Could you check a few things on this model? Use its own coordinates, in mm. Face numbers are marked on the shaded views. A direction names the side the tool comes from. Give positions to 0.01 mm unless a question says otherwise; leave off trailing zeros. Loops run counter-clockwise (first coordinate to the right, second up) from the corner with the lowest first, then second, coordinate; pieces in that order, holes last. Notation, with made-up numbers: (-28, 89) -> (11, 89) arc R13 ccw to (11, 96) -> close; hole circle Ø4 at (8.5, 11.25). An arc over 180 degrees is marked (long way). Write item = value, one per line. Start each with the question number.
1) I want a section at B-B (z = 3). List the corners of the cut face in (x, y) for me, and give its area (3 significant figures).
2) On a 3-axis mill with a long thin cutter (end or side, diameter ignored), from which of +Z, -Z, +X, -X, +Y, -Y can I reach the whole of each face in a straight line? I mean the marked faces 1, 2 and 3. Say none if no direction works.
3) I want a section at D-D (z = -32.5). List the corners of the cut face in (x, y) for me.
4) I want a section at A-A (y = -13). List the corners of the cut face in (x, z) for me.
5) I'm going to push flat-ended pins straight in: pin 1 Ø6 at (y, z) = (-9.5, -21.5) entering from +X; pin 2 Ø3 at (x, y) = (27, -13) entering from +Z; pin 3 Ø5 at (x, y) = (-2, -4) entering from +Z; pin 4 Ø4 at (x, z) = (4, -12) entering from +Y. Where does each tip first touch, or does it pass through?
6) If we mould it in two halves opening along X, with no side actions, what happens to the marked faces 4, 5 and 6? For each: +X half, -X half, draft (parallel to the pull), parting line (faces both ways), or undercut.
7) I need wall thicknesses on probe 1 along X at (y, z) = (-1.75, 7.5); probe 2 along Z at (x, y) = (-11, -0.5); probe 3 along Z at (x, y) = (2, -1.25). Which ranges of each line are inside material? Lowest first, please. Write a range as from..to.
8) I want a section at C-C (x = -2). List the corners of the cut face in (y, z) for me, and give its area (3 significant figures).
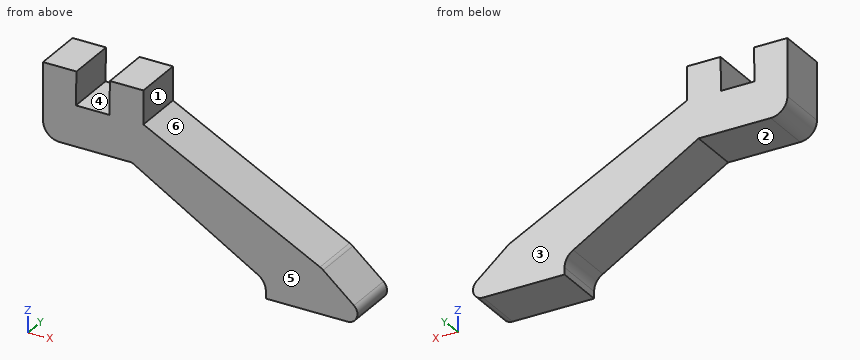
from build123d import *

# Parameters (mm, degrees)
F1_DEPTH = 15
F2_R     = 5


with BuildPart() as f1:
    # F0 (on Front) → F1 (new body)
    with BuildSketch(Plane.XZ):
        with BuildLine():
            Line((65.747503, -27.193502), (12.955731, 0))
            Line((12.955731, 0), (12.955731, 9.998409))
            Line((12.955731, 9.998409), (2.955731, 9.998409))
            Line((2.955731, 9.998409), (2.777357, 0))
            Line((2.777357, 0), (-7.222643, 0))
            Line((-7.222643, 0), (-7.044269, 9.998409))
            Line((-7.044269, 9.998409), (-17.044269, 9.998409))
            Line((-17.044269, 9.998409), (-17.044269, 0))
            Line((-17.044269, 0), (-17.044269, -12.098167))
            Line((-17.044269, -12.098167), (9.505874, -12.098167))
            Line((9.505874, -12.098167), (46.953158, -34.44976))
            ThreePointArc((46.953158, -34.44976), (48.861942, -36.287192), (49.563903, -38.841965))
            Line((49.563903, -38.841965), (49.563903, -40.925505))
            Line((49.563903, -40.925505), (73.922526, -40.925505))
            ThreePointArc((73.922526, -40.925505), (76.737769, -38.962041), (75.867925, -35.641776))
            Line((75.867925, -35.641776), (66.700202, -27.832236))
            ThreePointArc((66.700202, -27.832236), (66.242229, -27.48546), (65.747503, -27.193502))
        make_face()
    extrude(amount=F1_DEPTH)

    # F2
    f2_edges = [f1.edges().sort_by_distance(p)[0] for p in [
        (-17.044269, -7.5, -12.098167),
    ]]
    fillet(f2_edges, radius=F2_R)


solid = f1.part
Answer list:
q1.outline = (-17.04, -15) -> (-7.17, -15) -> (-7.17, 0) -> (-17.04, 0) -> close; (2.83, -15) -> (12.96, -15) -> (12.96, 0) -> (2.83, 0) -> close
q1.area = 300 mm^2
q2.face_1 = +Z, +X, +Y, -Y
q2.face_2 = -Z, -X, +Y, -Y
q2.face_3 = +Z, -Z, +X, -X, +Y
q3.outline = (43.69, -15) -> (72.18, -15) -> (72.18, 0) -> (43.69, 0) -> close
q4.outline = (-17.04, -7.1) arc R5 ccw to (-12.04, -12.1) -> (9.51, -12.1) -> (46.95, -34.45) arc R5 cw to (49.56, -38.84) -> (49.56, -40.93) -> (73.92, -40.93) arc R3 ccw to (75.87, -35.64) -> (66.7, -27.83) arc R5 ccw to (65.75, -27.19) -> (12.96, 0) -> (12.96, 10) -> (2.96, 10) -> (2.78, 0) -> (-7.22, 0) -> (-7.04, 10) -> (-17.04, 10) -> close
q5.pin_1 = 60.52
q5.pin_2 = -6.46
q5.pin_3 = 0
q5.pin_4 = 0
q6.face_4 = undercut
q6.face_5 = draft
q6.face_6 = +X half
q7.probe_1 = -17.04..-7.09, 2.91..12.96
q7.probe_2 = -12.1..10
q7.probe_3 = -12.1..0
q8.outline = (-15, -12.1) -> (0, -12.1) -> (0, 0) -> (-15, 0) -> close
q8.area = 181 mm^2
